```python
from build123d import *
from OCP.BRepFilletAPI import BRepFilletAPI_MakeChamfer

# Parameters (mm, degrees)
SKETCH1_W          = 403.606
SKETCH1_H          = 492.76
EXTRUDE1_DEPTH     = 6.35
FILLET1_R          = 15.748
FILLET2_R          = 3.81
SHELL1_T           = -1.6002
SKETCH4_R          = 2.0447
CUT_EXTRUDE2_DEPTH = 530.301320194
SKETCH5_R          = 2.0447
CUT_EXTRUDE4_DEPTH = 530.301320194
CHAMFER1_SIZE      = 0.8128
CHAMFER1_SIZE2     = 0.658192462


with BuildPart() as part:
    # Sketch1 → Extrude1 (new body)
    with BuildSketch(Plane(origin=(0, 0, 0), x_dir=(1, 0, 0), z_dir=(0, 1, 0))):
        with Locations((0, 242.9002)):
            Rectangle(SKETCH1_W, SKETCH1_H)
    extrude(amount=EXTRUDE1_DEPTH)

    # Fillet1
    fillet1_edges = [part.edges().sort_by_distance(p)[0] for p in [
        (-201.803, 3.175, -489.2802),
        (201.803, 3.175, -489.2802),
        (201.803, 3.175, 3.4798),
        (-201.803, 3.175, 3.4798),
    ]]
    fillet(fillet1_edges, radius=FILLET1_R)

    # Fillet2
    fillet2_edges = [part.edges().sort_by_distance(p)[0] for p in [
        (0, 0, 3.4798),
        (-201.803, 0, -242.9002),
        (0, 0, -489.2802),
        (201.803, 0, -242.9002),
        (197.19051759, 0, -1.13268241),
        (197.19051759, 0, -484.66771759),
        (-197.19051759, 0, -484.66771759),
        (-197.19051759, 0, -1.13268241),
    ]]
    fillet(fillet2_edges, radius=FILLET2_R)

    # Shell1
    shell1_openings = [part.faces().sort_by_distance(p)[0] for p in [
        (0, 6.35, -242.9002),
    ]]
    offset(amount=SHELL1_T, openings=shell1_openings, kind=Kind.INTERSECTION)

    # Sketch4 → Cut-Extrude2 (cut, through all)
    with BuildSketch(Plane(origin=(0, 0, 0), x_dir=(1, 0, 0), z_dir=(0, 1, 0))):
        with Locations(Location((183.134, 204.8002, 0), (0, 0, 270))):
            Circle(SKETCH4_R)
        with Locations(Location((0, 15.367, 0), (0, 0, 270))):
            Circle(SKETCH4_R)
        with Locations(Location((183.134, 128.6002, 0), (0, 0, 270))):
            Circle(SKETCH4_R)
        with Locations(Location((183.134, 433.4002, 0), (0, 0, 270))):
            Circle(SKETCH4_R)
        with Locations(Location((183.134, 281.0002, 0), (0, 0, 270))):
            Circle(SKETCH4_R)
        with Locations(Location((183.134, 357.2002, 0), (0, 0, 270))):
            Circle(SKETCH4_R)
        with Locations(Location((-183.134, 357.2002, 0), (0, 0, 90))):
            Circle(SKETCH4_R)
        with Locations(Location((-183.134, 281.0002, 0), (0, 0, 90))):
            Circle(SKETCH4_R)
        with Locations(Location((183.134, 52.4002, 0), (0, 0, 90))):
            Circle(SKETCH4_R)
        with Locations(Location((-183.134, 128.6002, 0), (0, 0, 90))):
            Circle(SKETCH4_R)
        with Locations(Location((-183.134, 204.8002, 0), (0, 0, 90))):
            Circle(SKETCH4_R)
        with Locations(Location((165.1, 15.367, 0), (0, 0, 270))):
            Circle(SKETCH4_R)
        with Locations(Location((-183.134, 52.4002, 0), (0, 0, 270))):
            Circle(SKETCH4_R)
        with Locations(Location((-183.134, 433.4002, 0), (0, 0, 90))):
            Circle(SKETCH4_R)
        with Locations(Location((-165.1, 470.4334, 0), (0, 0, 90))):
            Circle(SKETCH4_R)
        with Locations(Location((-76.2, 470.4334, 0), (0, 0, 90))):
            Circle(SKETCH4_R)
        with Locations(Location((76.2, 15.367, 0), (0, 0, 270))):
            Circle(SKETCH4_R)
        with Locations(Location((76.2, 470.4334, 0), (0, 0, 90))):
            Circle(SKETCH4_R)
        with Locations(Location((165.1, 470.4334, 0), (0, 0, 90))):
            Circle(SKETCH4_R)
        with Locations(Location((-76.2, 15.367, 0), (0, 0, 270))):
            Circle(SKETCH4_R)
        with Locations(Location((-165.1, 15.367, 0), (0, 0, 270))):
            Circle(SKETCH4_R)
        with Locations(Location((0, 470.4334, 0), (0, 0, 90))):
            Circle(SKETCH4_R)
    extrude(amount=CUT_EXTRUDE2_DEPTH, mode=Mode.SUBTRACT)

    # Sketch5 → Cut-Extrude4 (cut, through all)
    with BuildSketch(Plane(origin=(0, 0, 0), x_dir=(1, 0, 0), z_dir=(0, 1, 0))):
        with Locations(Location((122.6566, 6.1722, 0), (0, 0, 90))):
            Circle(SKETCH5_R)
        with Locations(Location((144.653, 6.1722, 0), (0, 0, 270))):
            Circle(SKETCH5_R)
        with Locations(Location((-122.6566, 6.1722, 0), (0, 0, 270))):
            Circle(SKETCH5_R)
        with Locations(Location((-144.653, 6.1722, 0), (0, 0, 90))):
            Circle(SKETCH5_R)
        with Locations(Location((-144.653, 479.6282, 0), (0, 0, 270))):
            Circle(SKETCH5_R)
        with Locations(Location((-122.6566, 479.6282, 0), (0, 0, 90))):
            Circle(SKETCH5_R)
        with Locations(Location((122.6566, 479.6282, 0), (0, 0, 270))):
            Circle(SKETCH5_R)
        with Locations(Location((144.653, 479.6282, 0), (0, 0, 90))):
            Circle(SKETCH5_R)
        with Locations(Location((-192.151, 231.902, 0), (0, 0, 270))):
            Circle(SKETCH5_R)
        with Locations(Location((-192.151, 253.8984, 0), (0, 0, 90))):
            Circle(SKETCH5_R)
        with Locations(Location((192.151, 253.8984, 0), (0, 0, 270))):
            Circle(SKETCH5_R)
        with Locations(Location((192.151, 231.902, 0), (0, 0, 90))):
            Circle(SKETCH5_R)
    extrude(amount=CUT_EXTRUDE4_DEPTH, mode=Mode.SUBTRACT)

    # Chamfer1: one chamfer whose edges measure the first distance from different faces: ONE call of the kernel's chamfer builder (chamfer() names one face for all edges)
    chamfer1_edges_1 = [part.edges().sort_by_distance(p)[0] for p in [
        (144.653, 1.6002, -8.2169),
    ]]
    chamfer1_side_1 = [part.faces().sort_by_distance(p)[0] for p in [
        (144.653, 0.8001, -8.2169),
    ]]
    chamfer1_edges_2 = [part.edges().sort_by_distance(p)[0] for p in [
        (122.6566, 1.6002, -4.1275),
    ]]
    chamfer1_side_2 = [part.faces().sort_by_distance(p)[0] for p in [
        (122.6566, 0.8001, -4.1275),
    ]]
    chamfer1_edges_3 = [part.edges().sort_by_distance(p)[0] for p in [
        (-122.6566, 1.6002, -8.2169),
    ]]
    chamfer1_side_3 = [part.faces().sort_by_distance(p)[0] for p in [
        (-122.6566, 0.8001, -8.2169),
    ]]
    chamfer1_edges_4 = [part.edges().sort_by_distance(p)[0] for p in [
        (-144.653, 1.6002, -4.1275),
    ]]
    chamfer1_side_4 = [part.faces().sort_by_distance(p)[0] for p in [
        (-144.653, 0.8001, -4.1275),
    ]]
    chamfer1_edges_5 = [part.edges().sort_by_distance(p)[0] for p in [
        (-144.653, 1.6002, -481.6729),
    ]]
    chamfer1_side_5 = [part.faces().sort_by_distance(p)[0] for p in [
        (-144.653, 0.8001, -481.6729),
    ]]
    chamfer1_edges_6 = [part.edges().sort_by_distance(p)[0] for p in [
        (-122.6566, 1.6002, -477.5835),
    ]]
    chamfer1_side_6 = [part.faces().sort_by_distance(p)[0] for p in [
        (-122.6566, 0.8001, -477.5835),
    ]]
    chamfer1_edges_7 = [part.edges().sort_by_distance(p)[0] for p in [
        (122.6566, 1.6002, -481.6729),
    ]]
    chamfer1_side_7 = [part.faces().sort_by_distance(p)[0] for p in [
        (122.6566, 0.8001, -481.6729),
    ]]
    chamfer1_edges_8 = [part.edges().sort_by_distance(p)[0] for p in [
        (144.653, 1.6002, -477.5835),
    ]]
    chamfer1_side_8 = [part.faces().sort_by_distance(p)[0] for p in [
        (144.653, 0.8001, -477.5835),
    ]]
    chamfer1_edges_9 = [part.edges().sort_by_distance(p)[0] for p in [
        (-192.151, 1.6002, -233.9467),
    ]]
    chamfer1_side_9 = [part.faces().sort_by_distance(p)[0] for p in [
        (-192.151, 0.8001, -233.9467),
    ]]
    chamfer1_edges_10 = [part.edges().sort_by_distance(p)[0] for p in [
        (-192.151, 1.6002, -251.8537),
    ]]
    chamfer1_side_10 = [part.faces().sort_by_distance(p)[0] for p in [
        (-192.151, 0.8001, -251.8537),
    ]]
    chamfer1_edges_11 = [part.edges().sort_by_distance(p)[0] for p in [
        (192.151, 1.6002, -255.9431),
    ]]
    chamfer1_side_11 = [part.faces().sort_by_distance(p)[0] for p in [
        (192.151, 0.8001, -255.9431),
    ]]
    chamfer1_edges_12 = [part.edges().sort_by_distance(p)[0] for p in [
        (192.151, 1.6002, -229.8573),
    ]]
    chamfer1_side_12 = [part.faces().sort_by_distance(p)[0] for p in [
        (192.151, 0.8001, -229.8573),
    ]]
    chamfer1 = BRepFilletAPI_MakeChamfer(part.part.solid().wrapped)
    for e in chamfer1_edges_1:
        chamfer1.Add(CHAMFER1_SIZE, CHAMFER1_SIZE2, e.wrapped, chamfer1_side_1[0].wrapped)  # the first distance lies on this face
    for e in chamfer1_edges_2:
        chamfer1.Add(CHAMFER1_SIZE, CHAMFER1_SIZE2, e.wrapped, chamfer1_side_2[0].wrapped)  # the first distance lies on this face
    for e in chamfer1_edges_3:
        chamfer1.Add(CHAMFER1_SIZE, CHAMFER1_SIZE2, e.wrapped, chamfer1_side_3[0].wrapped)  # the first distance lies on this face
    for e in chamfer1_edges_4:
        chamfer1.Add(CHAMFER1_SIZE, CHAMFER1_SIZE2, e.wrapped, chamfer1_side_4[0].wrapped)  # the first distance lies on this face
    for e in chamfer1_edges_5:
        chamfer1.Add(CHAMFER1_SIZE, CHAMFER1_SIZE2, e.wrapped, chamfer1_side_5[0].wrapped)  # the first distance lies on this face
    for e in chamfer1_edges_6:
        chamfer1.Add(CHAMFER1_SIZE, CHAMFER1_SIZE2, e.wrapped, chamfer1_side_6[0].wrapped)  # the first distance lies on this face
    for e in chamfer1_edges_7:
        chamfer1.Add(CHAMFER1_SIZE, CHAMFER1_SIZE2, e.wrapped, chamfer1_side_7[0].wrapped)  # the first distance lies on this face
    for e in chamfer1_edges_8:
        chamfer1.Add(CHAMFER1_SIZE, CHAMFER1_SIZE2, e.wrapped, chamfer1_side_8[0].wrapped)  # the first distance lies on this face
    for e in chamfer1_edges_9:
        chamfer1.Add(CHAMFER1_SIZE, CHAMFER1_SIZE2, e.wrapped, chamfer1_side_9[0].wrapped)  # the first distance lies on this face
    for e in chamfer1_edges_10:
        chamfer1.Add(CHAMFER1_SIZE, CHAMFER1_SIZE2, e.wrapped, chamfer1_side_10[0].wrapped)  # the first distance lies on this face
    for e in chamfer1_edges_11:
        chamfer1.Add(CHAMFER1_SIZE, CHAMFER1_SIZE2, e.wrapped, chamfer1_side_11[0].wrapped)  # the first distance lies on this face
    for e in chamfer1_edges_12:
        chamfer1.Add(CHAMFER1_SIZE, CHAMFER1_SIZE2, e.wrapped, chamfer1_side_12[0].wrapped)  # the first distance lies on this face
    add(Compound.cast(chamfer1.Shape()), mode=Mode.REPLACE)


solid = part.part
```
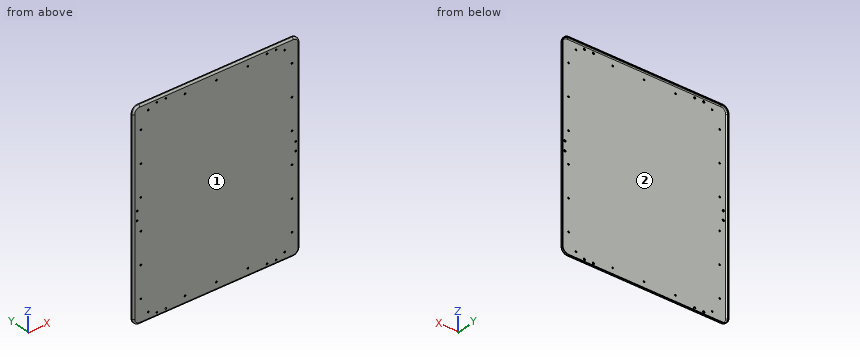
Work out the finished part from the listing and answer in its coordinate system (mm). Face numbers are marked on the shaded views. Give positions to 0.01 mm unless a question says otherwise; leave off trailing zeros. Loops run counter-clockwise (first coordinate to the right, second up) from the corner with the lowest first, then second, coordinate; pieces in that order, holes last. Notation, with made-up numbers: (10.5, 52.25) -> (34.5, 52.25) arc R20 cw to (34.5, 66.25) -> close; hole circle Ø4 at (18.5, -6.75). An arc over 180 degrees is marked (long way). Write item = value, one per line. Start each with the question number.
(1) Find the intervals of material crossed by probe 1 along Z at (x, y) = (76.2, 0.8); probe 2 along Z at (x, y) = (-76.2, 0.7); probe 3 along X at (y, z) = (4.5, -175.5), in increasing order. Write a range as from..to.
(2) Find section B-B on x = -20. Give the vertices of the cut face in (y, z), and give its area (3 significant figures).
(3) Find section A-A on z = -350. Give the vertices of the cut face in (x, y), and give its area (3 significant figures).
(4) Given pin 1 Ø2.5 at (x, z) = (76.2, -470.43) entering from +Y; pin 2 Ø8 at (x, z) = (-146, -282.5) entering from +Y; pin 3 Ø5.5 at (x, z) = (-192.151, -231.902) entering from -Y, each flat-ended and moving along its own axis, determine where each tip first touches the part or whether it passes through.
(5) The mould has two halves that part along Z. Classify the marked faces 1 and 2: +Z half, -Z half, draft (parallel to the pull), parting line (faces both ways), or undercut.
From the geometry:
q1.probe_1 = -487.81..-472.48, -468.39..-17.41, -13.32..2.01
q1.probe_2 = -487.67..-472.48, -468.39..-17.41, -13.32..1.87
q1.probe_3 = -201.8..-200.2, 200.2..201.8
q2.outline = (0, -485.47) arc R3.81 ccw to (3.81, -489.28) -> (6.35, -489.28) -> (6.35, -487.68) -> (3.81, -487.68) arc R2.21 cw to (1.6, -485.47) -> (1.6, -0.33) arc R2.21 cw to (3.81, 1.88) -> (6.35, 1.88) -> (6.35, 3.48) -> (3.81, 3.48) arc R3.81 ccw to (0, -0.33) -> close
q2.area = 800 mm^2
q3.outline = (-201.8, 3.81) arc R3.81 ccw to (-197.99, 0) -> (197.99, 0) arc R3.81 ccw to (201.8, 3.81) -> (201.8, 6.35) -> (200.2, 6.35) -> (200.2, 3.81) arc R2.21 cw to (197.99, 1.6) -> (-197.99, 1.6) arc R2.21 cw to (-200.2, 3.81) -> (-200.2, 6.35) -> (-201.8, 6.35) -> close
q3.area = 657 mm^2
q4.pin_1 = through
q4.pin_2 = 1.6
q4.pin_3 = 0
q5.face_1 = draft
q5.face_2 = undercut
